Part print with two shaded views. Sizes in mm from the minimum x, y, z corner. A direction names the side the tool comes from. Round coordinates to 2 decimals unless told otherwise and drop trailing zeros. Write each loop counter-clockwise with the first axis right and the second up, starting at its lowest first coordinate (ties: lowest second). Pieces come first, ordered by that corner, then holes. Notation, with made-up numbers: (-31, -29) -> (9, -29) arc R34 cw to (9, 4) -> close; hole circle Ø7 at (-7.75, -35). An arc over 180 degrees is marked (long way). Return JSON: item names as keys, results as strings.
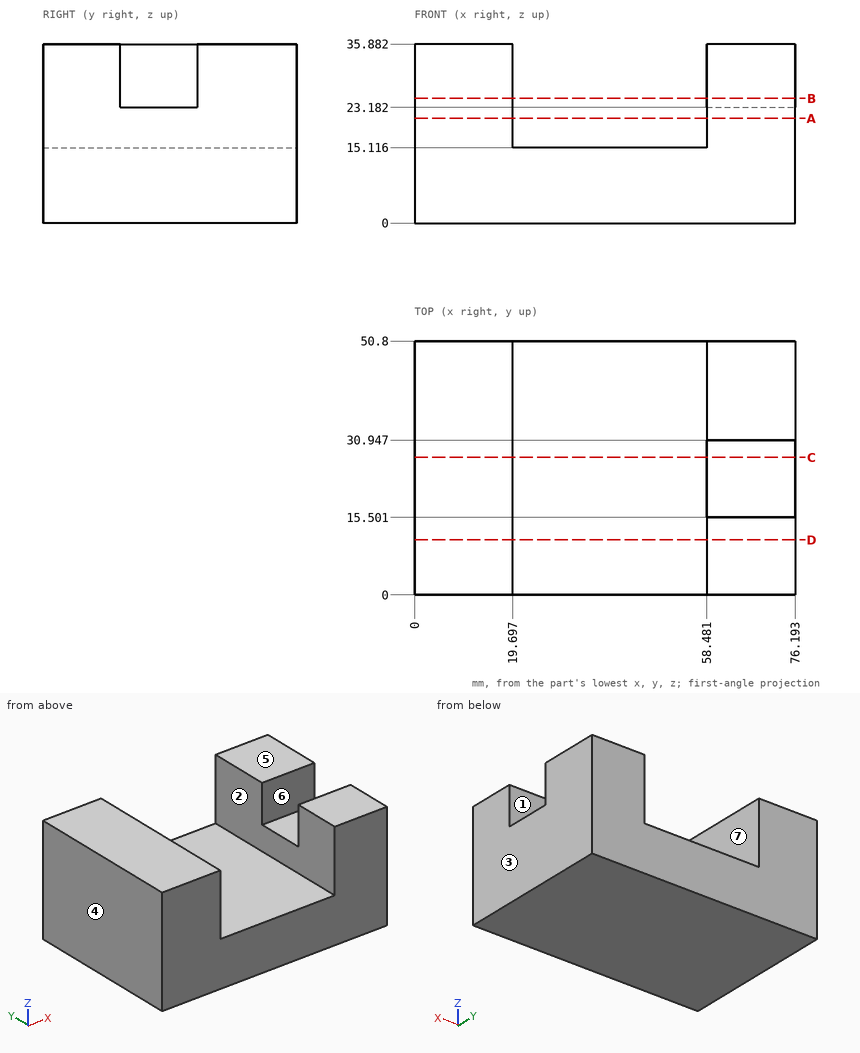
Q1. Saw through at D-D on y = 11. List the corners of the cut face in (x, z), then the cut area to 3 significant figures.
Verdict:
{"outline": "(0, 0) -> (76.19, 0) -> (76.19, 35.88) -> (58.48, 35.88) -> (58.48, 15.12) -> (19.7, 15.12) -> (19.7, 35.88) -> (0, 35.88) -> close", "area": "1,930 mm²"}
Q2. 3-axis set-ups, long thin cutter, end or side, ignore diameter. For the marked faces 5, 6 and 7: which of +Z, -Z, +X, -X, +Y, -Y reach the whole face in a straight line?
Verdict:
{"face 5": "+Z, +X, -X, +Y, -Y", "face 6": "+Z, +X", "face 7": "+Z, +Y, -Y"}
Q3. Saw through at C-C on y = 27.5. List the corners of the cut face in (x, z).
Verdict:
{"outline": "(0, 0) -> (76.19, 0) -> (76.19, 23.18) -> (58.48, 23.18) -> (58.48, 15.12) -> (19.7, 15.12) -> (19.7, 35.88) -> (0, 35.88) -> close"}
Q4. Wall check: L1, parallel to X at y = 45, z = 17; L2, parallel to Z at x = 37, y = 27; L3, parallel to X at y = 27, z = 34.5. Give the ranges that are in metal, low to high.
Verdict:
{"L1": "x = 0 to 19.7, 58.48 to 76.19", "L2": "z = 0 to 15.12", "L3": "x = 0 to 19.7"}
Q5. Saw through at A-A on z = 21. List the corners of the cut face in (x, y).
Verdict:
{"outline": "(0, 0) -> (19.7, 0) -> (19.7, 50.8) -> (0, 50.8) -> close; (58.48, 0) -> (76.19, 0) -> (76.19, 50.8) -> (58.48, 50.8) -> close"}
Q6. Two-plate mould, pull along X, no slides. Class the marked faces 1, 2, 3 and 4: +X half, -X half, draft (parallel to the pull), parting line (faces both ways), or undercut.
Verdict:
{"face 1": "draft", "face 2": "undercut", "face 3": "+X half", "face 4": "-X half"}
Q7. Pin check, flat tips, straight feed: pin 1 Ø7.5 at (x, y) = (71, 25.5) entering from +Z; pin 2 Ø3 at (x, y) = (21.5, 12) entering from +Z. Stop position of each tip, or through.
Verdict:
{"pin 1": "stops at z = 23.18", "pin 2": "stops at z = 15.12"}
Q8. Saw through at B-B on z = 25. List the corners of the cut face in (x, y).
Verdict:
{"outline": "(0, 0) -> (19.7, 0) -> (19.7, 50.8) -> (0, 50.8) -> close; (58.48, 0) -> (76.19, 0) -> (76.19, 15.5) -> (58.48, 15.5) -> close; (58.48, 30.95) -> (76.19, 30.95) -> (76.19, 50.8) -> (58.48, 50.8) -> close"}
